The model under review builds one solid part; all positions refer to its coordinate system, in mm. A direction names the side the tool comes from. Coordinates: 2 decimals unless noted, no trailing zeros. Order: outer loops, then holes, each group sorted by start corner. A loop starts at its lowest first (then second) coordinate and runs counter-clockwise, first axis right, second up. Notation, with made-up numbers: M -2,67 L 36,67 A12 ccw 36,87 Z; hole C 0,-27.75 d11. An arc over 180 degrees is marked long. One line per item, written item: value.
```python
from build123d import *

# Parameters (mm, degrees)
F0_R      = 15
F1_DEPTH  = 15
F2_W      = 15
F2_H      = 15
F3_DEPTH  = 20
F4_W      = 10.4
F4_H      = 10.4
F5_DEPTH  = 5
F7_START  = -1
F6_R      = 13.8
F7_DEPTH  = 13
F8_R      = 10.3
F9_DEPTH  = 2
F11_START = -2.3
F11_DEPTH = 10.4


with BuildPart() as f1:
    # F0 (on Top) → F1 (new body)
    with BuildSketch(Plane.XY):
        Circle(F0_R)
    extrude(amount=F1_DEPTH)

    # F2 (on Front) → F3 (join)
    with BuildSketch(Plane.XZ):
        with Locations((0, 7.5)):
            Rectangle(F2_W, F2_H)
    extrude(amount=F3_DEPTH)

    # F4 (on face) → F5 (cut)
    with BuildSketch(Plane.XZ.offset(20)):
        with Locations((0, 7.5)):
            Rectangle(F4_W, F4_H)
    extrude(amount=-F5_DEPTH, mode=Mode.SUBTRACT)

    # F6 (on face) → F7 (cut)
    with BuildSketch(Plane.XY.offset(15).offset(F7_START)):
        Circle(F6_R)
    extrude(amount=-F7_DEPTH, mode=Mode.SUBTRACT)

    # F8 (on face) → F9 (cut)
    with BuildSketch(Plane.XY.offset(15)):
        Circle(F8_R)
    extrude(amount=-F9_DEPTH, mode=Mode.SUBTRACT)

    # F10 (on face) → F11 (cut)
    with BuildSketch(Plane.XY.offset(15).offset(F11_START)):
        with BuildLine():
            Line((5.2, 8.8910066922), (5.2, 14.0698258696))
            ThreePointArc((5.2, 14.0698258696), (0, 15), (-5.2, 14.0698258696))
            Line((-5.2, 14.0698258696), (-5.2, 8.8910066922))
            ThreePointArc((-5.2, 8.8910066922), (0, 10.3), (5.2, 8.8910066922))
        make_face()
        with BuildLine():
            Line((8.8910066922, 5.2), (14.0698258696, 5.2))
            ThreePointArc((14.0698258696, 5.2), (10.6066017178, 10.6066017178), (5.2, 14.0698258696))
            Line((5.2, 14.0698258696), (5.2, 8.8910066922))
            ThreePointArc((5.2, 8.8910066922), (7.2831998462, 7.2831998462), (8.8910066922, 5.2))
        make_face()
        with BuildLine():
            Line((8.8910066922, -5.2), (14.0698258696, -5.2))
            ThreePointArc((14.0698258696, -5.2), (15, 0), (14.0698258696, 5.2))
            Line((14.0698258696, 5.2), (8.8910066922, 5.2))
            ThreePointArc((8.8910066922, 5.2), (9.9415131879, 2.6937549138), (10.3, 0))
            ThreePointArc((10.3, 0), (9.9415131879, -2.6937549138), (8.8910066922, -5.2))
        make_face()
    extrude(amount=-F11_DEPTH, mode=Mode.SUBTRACT)


solid = f1.part
```
(1) We need section C-C, the plane z = 5.5. State the section outline as (x, y) points, plus the area to 3 significant figures.
Geometry results:
outline: M -7.5,-20 L -5.2,-20 L -5.2,-15 L 5.2,-15 L 5.2,-20 L 7.5,-20 L 7.5,-12.99 A15 ccw 14.07,-5.2 L 12.78,-5.2 A13.8 cw long -5.2,12.78 L -5.2,14.07 A15 ccw -7.5,-12.99 Z
area: 101 mm2
(2) We need section A-A, the plane y = 0. State the section outline as (x, z) points, plus the area to 3 significant figures.
Geometry results:
outline: M -15,0 L 15,0 L 15,2.3 L 13.8,2.3 L 13.8,1 L -13.8,1 L -13.8,14 L -10.3,14 L -10.3,15 L -15,15 Z; M 10.3,14 L 13.8,14 L 13.8,12.7 L 15,12.7 L 15,15 L 10.3,15 Z
area: 58.1 mm2
(3) We need section D-D, the plane y = -12.5. State the section outline as (x, z) points.
Geometry results:
outline: M -8.29,0 L 8.29,0 L 8.29,15 L -8.29,15 Z; hole M -5.85,1 L 5.85,1 L 5.85,14 L -5.85,14 Z
(4) Tool access review of faces 5 (the flat face through (7.5, -16, 7)), 6 (the flat face through (0, 0, 1)), 7 (the flat face through (11, 9, 12.7)), 8 (the flat face through (0, -18, 2.3)): name each direction out of +Z, -Z, +X, -X, +Y, -Y from which nothing blocks a thin tool from reaching the whole face with its end or side.
Geometry results:
face 5: +Z, -Z, +X, -Y
face 6: none
face 7: +X, +Y
face 8: -Y
(5) Insertion check: pin 1 Ø5.5 at (y, z) = (-18, 7.5) entering from -X; pin 2 Ø3 at (x, z) = (-0.5, 5.5) entering from -Y; pin 3 Ø8 at (y, z) = (-9.5, 7) entering from +X. Each pin has a flat end and moves straight along its axis. Give the tip position at first contact, or say it passes through.
Geometry results:
pin 1: stops at x = -7.5
pin 2: stops at y = -15
pin 3: stops at x = 13.96
(6) We need section B-B, the plane x = 0. State the section outline as (y, z) points, plus the area to 3 significant figures.
Geometry results:
outline: M -20,0 L 15,0 L 15,2.3 L 13.8,2.3 L 13.8,1 L -13.8,1 L -13.8,14 L -10.3,14 L -10.3,15 L -20,15 L -20,12.7 L -15,12.7 L -15,2.3 L -20,2.3 Z; M 10.3,14 L 13.8,14 L 13.8,12.7 L 15,12.7 L 15,15 L 10.3,15 Z
area: 81.1 mm2
(7) For L1, parallel to Y at x = 0, z = 14.2; L2, parallel to Z at x = -6, y = -12; L3, parallel to Z at x = 3.25, y = 13.5, list the stretches that pass through material, from the lowest coordinate up.
Geometry results:
L1: y = -20 to -10.3, 10.3 to 15
L2: z = 0 to 1, 14 to 15
L3: z = 0 to 2.3, 12.7 to 15
(8) Mouldability with a two-part tool opening along Z and no side actions: class faces 1 (the cylindrical face through (-2.992, -13.472, 7.591)), 2 (the flat face through (0, -2, 0)), 3 (the flat face through (0, -18, 12.7)), 4 (the flat face through (-7, -20, 8)) as +Z half, -Z half, draft (parallel to the pull), parting line (faces both ways), or undercut.
Geometry results:
face 1: undercut
face 2: -Z half
face 3: undercut
face 4: draft
